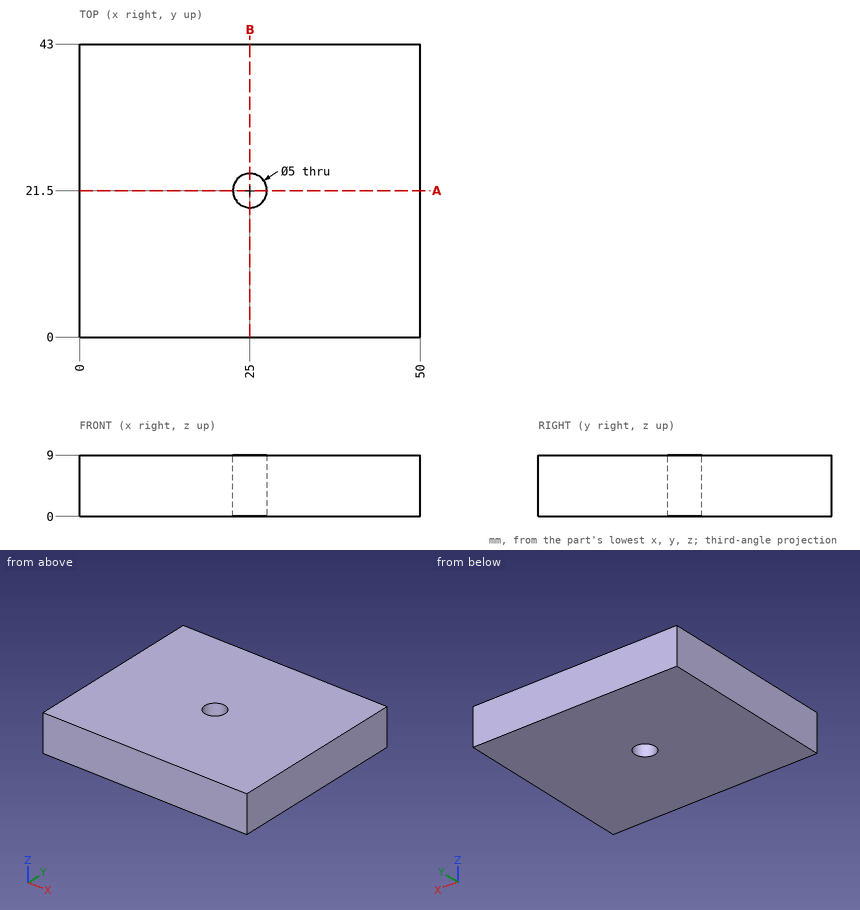
Check sheet for the drawn part. Datum: minimum x, y, z corner. Units: mm. Give positions to 0.01 mm unless a question says otherwise; leave off trailing zeros. Order: outer loops, then holes, each group sorted by start corner. A loop starts at its lowest first (then second) coordinate and runs counter-clockwise, first axis right, second up. Notation, with made-up numbers: (89, 53.25) - (147, 53.25) arc R28 cw to (147, 76.25) - close; hole circle Ø1 at (-15.5, -10). An arc over 180 degrees is marked (long way). Answer in a Markdown table with one row per item. Add a question column.
Q1. Cross-section at B-B, the plane x = 25. Enter the section's corners in (y, z).
Q2. Material ranges on probe 1 along Y at (x, z) = (25, 5.5); probe 2 along X at (y, z) = (21, 8); probe 3 along Y at (x, z) = (26.5, 0.5), recorded low to high. Write a range as from..to.
Q3. Cross-section at A-A, the plane y = 21.5. Enter the section's corners in (x, z), then the cut area to 3 significant figures.
Check values:
| question | item | result |
|---|---|---|
| 1 | outline | (0, 0) - (19, 0) - (19, 9) - (0, 9) - close; (24, 0) - (43, 0) - (43, 9) - (24, 9) - close |
| 2 | probe 1 | y = 0..19, 24..43 |
| 2 | probe 2 | x = 0..22.55, 27.45..50 |
| 2 | probe 3 | y = 0..19.5, 23.5..43 |
| 3 | outline | (0, 0) - (22.5, 0) - (22.5, 9) - (0, 9) - close; (27.5, 0) - (50, 0) - (50, 9) - (27.5, 9) - close |
| 3 | area | 405 mm^2 |
